Autodesk Inventor part; units mm, degrees
ref_plane "YZ Plane" through (0, 0, 0) normal (1, 0, 0) x (0, 1, 0)
ref_plane "XZ Plane" through (0, 0, 0) normal (0, 1, 0) x (-1, 0, 0)
ref_plane "XY Plane" through (0, 0, 0) normal (0, 0, 1) x (1, 0, 0)
sketch "Boceto1" plane through (0, 0, 0) normal (0, 1, 0) x (-1, 0, 0)
  arc A0 (14.5, 25.1147) -> (0, 29) centre (0, 0) ccw
  arc A1 (0, -189) -> (14.5, -185.1147) centre (0, -160) ccw
  line L0 (37, 0) -> (29, 0)
  line L1 (37, -35) -> (29, -35)
  line L2 (29, -65) -> (37, -65)
  line L3 (29, -95) -> (37, -95)
  line L4 (29, -125) -> (37, -125)
  line L5 (29, -160) -> (37, -160)
  line L6 (14.5, 25.1147) -> (18.5, 32.0429)
  line L7 (14.5, -185.1147) -> (18.5, -192.0429)
  line L8 (0, 62.7565) -> (0, -215.9435)
  arc A2 (37, 0) -> (18.5, 32.0429) centre (0, 0) ccw
  line L9 (29, 0) -> (29, -35)
  line L10 (37, -35) -> (37, -65)
  line L11 (37, -95) -> (37, -125)
  line L12 (29, -65) -> (29, -95)
  line L13 (29, -125) -> (29, -160)
  arc A3 (18.5, -192.0429) -> (37, -160) centre (0, -160) ccw
  arc A4 (0, 29) -> (-14.5, 25.1147) centre (0, 0) ccw
  arc A5 (-14.5, -185.1147) -> (0, -189) centre (0, -160) ccw
  line L14 (-37, 0) -> (-29, 0)
  line L15 (-37, -35) -> (-29, -35)
  line L16 (-29, -65) -> (-37, -65)
  line L17 (-29, -95) -> (-37, -95)
  line L18 (-29, -125) -> (-37, -125)
  line L19 (-29, -160) -> (-37, -160)
  line L20 (-14.5, 25.1147) -> (-18.5, 32.0429)
  line L21 (-14.5, -185.1147) -> (-18.5, -192.0429)
  arc A6 (-18.5, 32.0429) -> (-37, 0) centre (0, 0) ccw
  line L22 (-29, 0) -> (-29, -35)
  line L23 (-37, -35) -> (-37, -65)
  line L24 (-37, -95) -> (-37, -125)
  line L25 (-29, -65) -> (-29, -95)
  line L26 (-29, -125) -> (-29, -160)
  arc A7 (-37, -160) -> (-18.5, -192.0429) centre (0, -160) ccw
  dimension "d1" = 58
  dimension "d3" = 58
  dimension "d4" = 160
  dimension "d5" = 35
  dimension "d6" = 30
  dimension "d7" = 30
  dimension "d8" = 30
  dimension "d9" = 35
  dimension "d10" = 60
  dimension "d11" = 60
extrude "Extrusión1" add sketch "Boceto1" along normal blind 7
sketch "Boceto2" plane through (0, 7, 0) normal (0, 1, 0) x (1, 0, 0)
  circle A0 centre (-33, 50) radius 2.05
  circle A1 centre (-33, 110) radius 2.05
  arc A2 (-18.5, 192.0429) -> (-37, 160) centre (0, 160) ccw
  circle A3 centre (0, 160) radius 33
  circle A4 centre (0, 0) radius 33
  circle A5 centre (-21.212, -25.2795) radius 2.05
  line L0 (0, -60.8488) -> (0, 208.5153)
  circle A6 centre (-28.5788, 176.5) radius 2.05
  line L1 (-29, 65) -> (-37, 65)
  line L2 (-37, 65) -> (-37, 35)
  line L3 (-29, 125) -> (-37, 125)
  line L4 (-37, 125) -> (-37, 95)
  line L5 (-28.5788, 176.5) -> (0, 160)
  line L6 (0, 0) -> (-21.212, -25.2795)
  line L7 (-29, 0) -> (-37, 0)
  line L8 (-37, 160) -> (-29, 160)
  circle A7 centre (33, 50) radius 2.05
  circle A8 centre (33, 110) radius 2.05
  circle A9 centre (21.212, -25.2795) radius 2.05
  circle A10 centre (28.5788, 176.5) radius 2.05
  dimension "d14" = 66
  dimension "d15" = 66
  dimension "d16" = 4.1
  dimension "d17" = 15
  dimension "d18" = 4
  dimension "d19" = 15
  dimension "d20" = 4
  dimension "d21" = 50
  dimension "d22" = 30
extrude "Extrusión2" cut sketch "Boceto2" against normal through all contours A0 | A1 | A10 A3 | A3 A10 | A6 A3 | A3 L5 A6 | L5 A3 A6 | A9 A4 | A4 A9 | A5 L6 A4 | A4 A5 | A5 A4 L6 | A7 | A8
sketch "Boceto3" plane through (0, 7, 0) normal (0, 1, 0) x (1, 0, 0)
  circle A0 centre (-33, 50) radius 2.05
  circle A1 centre (-33, 50) radius 3
  circle A2 centre (-33, 110) radius 2.05
  circle A3 centre (-33, 110) radius 3
  circle A4 centre (-28.5788, 176.5) radius 2.05
  circle A5 centre (-28.5788, 176.5) radius 3
  circle A6 centre (-21.212, -25.2795) radius 2.05
  circle A7 centre (-21.212, -25.2795) radius 3
  line L0 (0, -43.6501) -> (0, 201.1209)
  circle A8 centre (33, 50) radius 2.05
  circle A9 centre (33, 50) radius 3
  circle A10 centre (33, 110) radius 2.05
  circle A11 centre (33, 110) radius 3
  circle A12 centre (28.5788, 176.5) radius 2.05
  circle A13 centre (28.5788, 176.5) radius 3
  circle A14 centre (21.212, -25.2795) radius 2.05
  circle A15 centre (21.212, -25.2795) radius 3
  point P0 (0, 0)
  dimension "d25" = 6
extrude "Extrusión3" cut sketch "Boceto3" against normal blind 3 contours A0 | A1 | A2 | A3 | A4 | A5 | A6 | A7 | A8 | A9 | A10 | A11 | A12 | A13 | A14 | A15
sketch "Boceto4" plane through (0, 7, 0) normal (0, 1, 0) x (1, 0, 0)
  arc A0 (14.5, 185.1147) -> (-14.5, 185.1147) centre (0, 160) ccw
  arc A1 (-18.5, 192.0429) -> (-37, 160) centre (0, 160) ccw
  circle A2 centre (0, 160) radius 11
  circle A3 centre (0, 64) radius 11
  line L0 (0, 12.5) -> (0, 19.5) construction
  line L1 (11.1, 12.5) -> (11.1, 19.5)
  line L2 (-11.1, 19.5) -> (-11.1, 12.5)
  arc A4 (-11.1, 12.5) -> (11.1, 12.5) centre (0, 12.5) ccw
  arc A5 (11.1, 19.5) -> (-11.1, 19.5) centre (0, 19.5) ccw
  line L3 (-15.5, -3) -> (-15.5, 4) construction
  line L4 (-13.95, -3) -> (-13.95, 4)
  line L5 (-17.05, 4) -> (-17.05, -3)
  arc A6 (-17.05, -3) -> (-13.95, -3) centre (-15.5, -3) ccw
  arc A7 (-13.95, 4) -> (-17.05, 4) centre (-15.5, 4) ccw
  line L6 (4.1829, 16) -> (-3.8668, 16)
  line L7 (0, 6.9157) -> (0, 25.6477)
  line L8 (-15.5, 35) -> (-15.5, 28) construction
  line L9 (-13.95, 35) -> (-13.95, 28)
  line L10 (-17.05, 28) -> (-17.05, 35)
  arc A8 (-13.95, 35) -> (-17.05, 35) centre (-15.5, 35) ccw
  arc A9 (-17.05, 28) -> (-13.95, 28) centre (-15.5, 28) ccw
  line L11 (15.5, -3) -> (15.5, 4) construction
  line L12 (13.95, -3) -> (13.95, 4)
  line L13 (17.05, 4) -> (17.05, -3)
  arc A10 (13.95, -3) -> (17.05, -3) centre (15.5, -3) ccw
  arc A11 (17.05, 4) -> (13.95, 4) centre (15.5, 4) ccw
  arc A12 (13.95, 28) -> (17.05, 28) centre (15.5, 28) ccw
  line L14 (13.95, 35) -> (13.95, 28)
  line L15 (15.5, 35) -> (15.5, 28) construction
  arc A13 (17.05, 35) -> (13.95, 35) centre (15.5, 35) ccw
  line L16 (17.05, 28) -> (17.05, 35)
  point P0 (0, 189)
  point P1 (0, 16)
  point P2 (-15.5, 0.5)
  point P3 (-15.5, 31.5)
  point P4 (15.5, 0.5)
  point P5 (15.5, 31.5)
  dimension "d37" = 22
  dimension "d38" = 96
  dimension "d41" = 22.2
  dimension "d42" = 7
  dimension "d43" = 44.5
  dimension "d44" = 3.1
  dimension "d45" = 7
  dimension "d46" = 15.5
  dimension "d47" = 15.5
extrude "Extrusión4" cut sketch "Boceto4" against normal through all
sketch "Boceto7" plane through (0, 7, 0) normal (0, 1, 0) x (1, 0, 0)
  line L0 (-29, 65) -> (-37, 65)
  line L1 (-37, 65) -> (-29, 65)
  line L2 (-29, 65) -> (-29, 64.8)
  line L3 (-29, 64.8) -> (-37, 64.8)
  line L4 (-37, 64.8) -> (-37, 65)
  line L5 (-37, 35) -> (-29, 35)
  line L6 (-37, 35) -> (-29, 35)
  line L7 (-29, 35) -> (-29, 35.2)
  line L8 (-29, 35.2) -> (-37, 35.2)
  line L9 (-37, 35.2) -> (-37, 35)
  line L10 (-37, 125) -> (-37, 95)
  line L11 (-37, 95) -> (-29, 95)
  line L12 (-29, 95) -> (-29, 95.2)
  line L13 (-29, 95.2) -> (-37, 95.2)
  line L14 (-37, 95.2) -> (-37, 95)
  line L15 (-37, 125) -> (-29, 125)
  line L16 (-29, 125) -> (-29, 124.8)
  line L17 (-29, 124.8) -> (-37, 124.8)
  line L18 (-37, 124.8) -> (-37, 125)
  line L19 (-37, 160) -> (-29, 160)
  line L20 (-37, 160) -> (-29, 160)
  line L21 (-29, 160) -> (-29, 160.2)
  line L22 (-29, 160.2) -> (-37, 160.2)
  line L23 (-37, 160.2) -> (-37, 160)
  line L24 (-29, 0) -> (-37, 0)
  line L25 (-37, 0) -> (-29, 0)
  line L26 (-29, 0) -> (-29, -0.2)
  line L27 (-29, -0.2) -> (-37, -0.2)
  line L28 (-37, -0.2) -> (-37, 0)
  line L29 (-14.5, 185.1147) -> (-18.5, 192.0429)
  line L30 (-14.5, 185.1147) -> (-14.6732, 185.0147)
  line L31 (-14.6732, 185.0147) -> (-18.6732, 191.9429)
  arc A0 (-18.5, 192.0429) -> (-37, 160) centre (0, 160) ccw
  line L32 (-18.6732, 191.9429) -> (-18.5, 192.0429)
  line L33 (-18.5, -32.0429) -> (-14.5, -25.1147)
  line L34 (-14.5, -25.1147) -> (-14.6732, -25.0147)
  line L35 (-14.6732, -25.0147) -> (-18.6732, -31.9429)
  arc A1 (-37, 0) -> (-18.5, -32.0429) centre (0, 0) ccw
  line L36 (-18.6732, -31.9429) -> (-18.5, -32.0429)
  line L37 (0, 208.262) -> (0, -50.4937)
  line L38 (29, 65) -> (37, 65)
  line L39 (37, 65) -> (29, 65)
  line L40 (29, 65) -> (29, 64.8)
  line L41 (29, 64.8) -> (37, 64.8)
  line L42 (37, 64.8) -> (37, 65)
  line L43 (37, 35) -> (29, 35)
  line L44 (37, 35) -> (29, 35)
  line L45 (29, 35) -> (29, 35.2)
  line L46 (29, 35.2) -> (37, 35.2)
  line L47 (37, 35.2) -> (37, 35)
  line L48 (37, 125) -> (37, 95)
  line L49 (37, 95) -> (29, 95)
  line L50 (29, 95) -> (29, 95.2)
  line L51 (29, 95.2) -> (37, 95.2)
  line L52 (37, 95.2) -> (37, 95)
  line L53 (37, 125) -> (29, 125)
  line L54 (29, 125) -> (29, 124.8)
  line L55 (29, 124.8) -> (37, 124.8)
  line L56 (37, 124.8) -> (37, 125)
  line L57 (37, 160) -> (29, 160)
  line L58 (37, 160) -> (29, 160)
  line L59 (29, 160) -> (29, 160.2)
  line L60 (29, 160.2) -> (37, 160.2)
  line L61 (37, 160.2) -> (37, 160)
  line L62 (29, 0) -> (37, 0)
  line L63 (37, 0) -> (29, 0)
  line L64 (29, 0) -> (29, -0.2)
  line L65 (29, -0.2) -> (37, -0.2)
  line L66 (37, -0.2) -> (37, 0)
  line L67 (14.5, 185.1147) -> (18.5, 192.0429)
  line L68 (14.5, 185.1147) -> (14.6732, 185.0147)
  line L69 (14.6732, 185.0147) -> (18.6732, 191.9429)
  arc A2 (37, 160) -> (18.5, 192.0429) centre (0, 160) ccw
  line L70 (18.6732, 191.9429) -> (18.5, 192.0429)
  line L71 (18.5, -32.0429) -> (14.5, -25.1147)
  line L72 (14.5, -25.1147) -> (14.6732, -25.0147)
  line L73 (14.6732, -25.0147) -> (18.6732, -31.9429)
  arc A3 (18.5, -32.0429) -> (37, 0) centre (0, 0) ccw
  line L74 (18.6732, -31.9429) -> (18.5, -32.0429)
  point P0 (-36.9995, -0.2)
  point P1 (-36.9995, 160.2)
  point P2 (-18.6729, 191.9425)
  point P3 (18.6729, 191.9425)
  point P4 (36.9995, 160.2)
  point P5 (36.9995, -0.2)
  point P6 (18.6729, -31.9425)
  dimension "d66" = 0.2
extrude "Extrusión7" cut sketch "Boceto7" against normal through all
properties part number "Segundo segmento - superior" material "Plastico PETG"
Geometry check sheet. Reference: the model listing, model coordinates, mm. A direction names the side the tool comes from. Round coordinates to 2 decimals unless told otherwise and drop trailing zeros. Loops run counter-clockwise (first coordinate to the right, second up) from the corner with the lowest first, then second, coordinate; pieces in that order, holes last.
Item 1: Cross-section at A-A on x = 5. Record the boundary of the cut face in (y, z), then the cut area to 3 significant figures.
Item 2: Access from +Z, -Z, +X, -X, +Y, -Y to the whole of each face (thin tool, end or side, straight path). Record for faces 4 (the flat face through (33, 4, -160.2)), 5 (the flat face through (-31, 4, -109)), 6 (the flat face through (-29, 4, -18)).
Item 3: Mould release check, pull along X, two halves, no side actions. Record for faces 1 (the flat face through (33, 4, 0.2)), 2 (the cylindrical face through (32.176, 3.451, 18.267)), 3 (the cylindrical face through (30, 6, -110)): pulls with the +X half, pulls with the -X half, needs draft (parallel to the pull), parting line crosses it, or undercut.
Item 4: Thickness scan on line 1 (X direction, y = 2.8, z = -50); line 2 (X direction, y = 5.85, z = -50); line 3 (Z direction, x = -0.5, y = 5). Record the ranges inside material, lowest first.
Item 5: Cross-section at C-C on x = -8. Record the boundary of the cut face in (y, z), then the cut area to 3 significant figures.
Item 6: Cross-section at D-D on y = 2.75. Count the separate pieces of the cut face and the enclosed holes in it, then the cut area to 3 significant figures.
Item 7: Cross-section at B-B on z = -176.5. Record the boundary of the cut face in (x, y), then the cut area to 3 significant figures.
Item 8: Gauge pin test, flat ends, axial feed: pin 1 (2 mm diameter, centred on y = 4.5, z = -32, fed in from +X); pin 2 (5.5 mm diameter, centred on x = 28.58, z = -176.5, fed in from -Y); pin 3 (2 mm diameter, centred on y = 3, z = -152.5, fed in from -X); pin 4 (5.5 mm diameter, centred on x = -28.58, z = -176.5, fed in from +Y). Record the tip position at first contact, or that the pin passes through.
Answer sheet:
1. outline: (0, -188.57) - (7, -188.57) - (7, -169.8) - (0, -169.8) - close; (0, -150.2) - (7, -150.2) - (7, -73.8) - (0, -73.8) - close; (0, -54.2) - (7, -54.2) - (7, -29.41) - (0, -29.41) - close; (0, -2.59) - (7, -2.59) - (7, 28.57) - (0, 28.57) - close
1. area: 1,060 mm2
2. face 4: +X, +Y, -Y
2. face 5: +Y
2. face 6: -X, +Y, -Y
3. face 1: needs draft
3. face 2: pulls with the +X half
3. face 3: undercut
4. line 1: x = -37 to -35.05, -30.95 to 30.95, 35.05 to 37
4. line 2: x = -37 to -36, -30 to 30, 36 to 37
4. line 3: z = -189 to -170.99, -149.01 to -74.99, -53.01 to -30.59, -1.41 to 29
5. outline: (0, -187.87) - (7, -187.87) - (7, -167.55) - (0, -167.55) - close; (0, -152.45) - (7, -152.45) - (7, -71.55) - (0, -71.55) - close; (0, -56.45) - (7, -56.45) - (7, -27.19) - (0, -27.19) - close; (0, -4.81) - (7, -4.81) - (7, 27.87) - (0, 27.87) - close
5. area: 1,140 mm2
6. separate pieces: 1
6. enclosed holes: 15
6. area: 12,400 mm2
7. outline: (-33.12, 0) - (-30.63, 0) - (-30.63, 4) - (-31.58, 4) - (-31.58, 7) - (-33.12, 7) - close; (-26.53, 0) - (26.53, 0) - (26.53, 4) - (25.58, 4) - (25.58, 7) - (-25.58, 7) - (-25.58, 4) - (-26.53, 4) - close; (30.63, 0) - (33.12, 0) - (33.12, 7) - (31.58, 7) - (31.58, 4) - (30.63, 4) - close
7. area: 395 mm2
8. pin 1: stops at x = 29
8. pin 2: stops at y = 0
8. pin 3: stops at x = -29
8. pin 4: stops at y = 4
